The listing builds one solid part. Answer for the finished solid, in the listing's coordinates (mm). Face numbers are marked on the shaded views. Round coordinates to 2 decimals unless told otherwise and drop trailing zeros. Order: outer loops, then holes, each group sorted by start corner. A loop starts at its lowest first (then second) coordinate and runs counter-clockwise, first axis right, second up. Notation, with made-up numbers: (-39, 29.25) -> (-31, 29.25) arc R19 cw to (-31, 49.25) -> close; hole circle Ø11 at (36, -2). An arc over 180 degrees is marked (long way). Return JSON: item names as keys, results as strings. Group by question number.
(1) Each of these flat-tipped pins is pushed along its axis until it touches: pin 1 (2 mm diameter, centred on x = 0, y = 3, fed in from +Z); pin 2 (2.5 mm diameter, centred on x = -22.65, z = 16.46, fed in from -Y); pin 3 (5 mm diameter, centred on x = 19.02, z = 6.18, fed in from -Y); pin 4 (3 mm diameter, centred on x = -9, z = -26, fed in from -Y). Where does it stop, or does it pass through?
(2) The part is cut by section A-A (x = 0). Determine the outline of the cut face in (y, z), plus the area to 3 significant figures.
(3) Consider line 1 (Z direction, x = 0, y = 6.8); line 2 (Z direction, x = 23, y = 0.5); line 3 (X direction, y = 1, z = 25.5). Determine where each line is inside the solid, lowest interval first. Write a range as [from, to].
(4) The part is cut by section B-B (z = 0). Determine the outline of the cut face in (x, y), plus the area to 3 significant figures.
(5) Determine the mould class of the marked faces 1, 2 and 3 for opening direction X: +X half, -X half, draft (parallel to the pull), parting line (faces both ways), or undercut.
(6) The part is cut by section C-C (x = 28). Determine the outline of the cut face in (y, z), plus the area to 3 significant figures.
(7) The part is cut by section D-D (z = -8). Determine the outline of the cut face in (x, y).
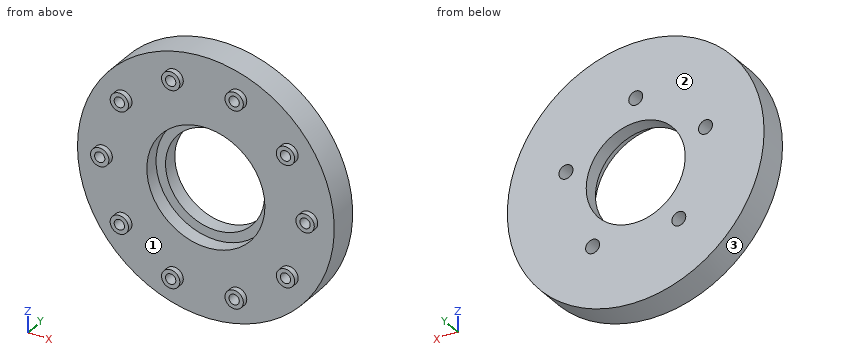
Autodesk Inventor part; units mm, degrees
ref_plane "YZ Plane" through (0, 0, 0) normal (1, 0, 0) x (0, 1, 0)
ref_plane "XZ Plane" through (0, 0, 0) normal (0, 1, 0) x (-1, 0, 0)
ref_plane "XY Plane" through (0, 0, 0) normal (0, 0, 1) x (1, 0, 0)
sketch "Szkic1" plane through (0, 0, 0) normal (0, 1, 0) x (-1, 0, 0)
  circle A0 centre (0, 0) radius 35
  dimension "d0" = 70
extrude "Wyciągnięcie proste1" add sketch "Szkic1" along normal blind 8
sketch "Szkic2" plane through (0, 0, 0) normal (0, -1, 0) x (1, 0, 0)
  circle A0 centre (0, 0) radius 28
  circle A1 centre (28, 0) radius 2.5
  dimension "d3" = 56
  dimension "d4" = 5
sketch "Szkic3" plane through (0, 0, 0) normal (0, -1, 0) x (1, 0, 0)
  circle A0 centre (0, 0) radius 16.1
  dimension "d9" = 32.2
extrude "Wyciągnięcie proste2" cut sketch "Szkic3" against normal blind 4
extrude "Wyciągnięcie proste3" add sketch "Szkic2" along normal blind 1.5 contours A0 A1 | A0 A1 picked at (27.2137, -0.5653) picked at (28.742, -0.6489)
pattern_circular "Szyk kołowy1" count 10 over 360 about axis through (0, 0, 0) along (0, 1, 0) of "Wyciągnięcie proste3"
sketch "Szkic4" plane through (0, 4, 0) normal (0, -1, 0) x (1, 0, 0)
  circle A0 centre (0, 0) radius 13.5
  dimension "d17" = 27
extrude "Wyciągnięcie proste4" cut sketch "Szkic4" against normal blind 4
sketch "Szkic5" plane through (28, -1.5, 0) normal (0, -1, 0) x (1, 0, 0)
  circle A0 centre (0, 0) radius 2.5
  circle A1 centre (0, 0) radius 1.4
  point P0 (-28, 0)
  dimension "d20" = 2.8
extrude "Wyciągnięcie proste5" cut sketch "Szkic5" against normal blind 6 contours A1
pattern_circular "Szyk kołowy2" count 10 over 360 about axis through (0, 0, 0) along (0, 1, 0) of "Wyciągnięcie proste5"
sketch "Szkic6" plane through (0, 8, 0) normal (0, 1, 0) x (1, 0, 0)
  circle A0 centre (0, 0) radius 20
  circle A1 centre (0, -20) radius 1.9
  dimension "d26" = 40
  dimension "d27" = 3.8
extrude "Wyciągnięcie proste6" cut sketch "Szkic6" against normal blind 6 contours A1 A0 | A0 A1 picked at (0.074, -19.3643) picked at (0.0625, -20.6235)
pattern_circular "Szyk kołowy3" count 5 over 360 about axis through (0, 4, 0) along (0, 1, 0) of "Wyciągnięcie proste6"
properties part number "_Drukowanie 3D"
Answer below:
{
 "1": {"pin 1": "stops at z = 35", "pin 2": "stops at y = 4.5", "pin 3": "stops at y = 0", "pin 4": "stops at y = -1.5"},
 "2": {"outline": "(0, -35) -> (8, -35) -> (8, -13.5) -> (4, -13.5) -> (4, -16.1) -> (0, -16.1) -> close; (0, 16.1) -> (4, 16.1) -> (4, 13.5) -> (8, 13.5) -> (8, 18.1) -> (2, 18.1) -> (2, 21.9) -> (8, 21.9) -> (8, 35) -> (0, 35) -> close", "area": "300 mm²"},
 "3": {"line 1": "z = [-35, -13.5], [13.5, 18.1], [21.9, 35]", "line 2": "z = [-26.38, -17.81], [-15.1, 15.1], [17.81, 26.38]", "line 3": "x = [-23.97, -9.48], [-7.83, 7.83], [9.48, 23.97]"},
 "4": {"outline": "(-35, 0) -> (-30.5, 0) -> (-30.5, -1.5) -> (-29.4, -1.5) -> (-29.4, 4.5) -> (-26.6, 4.5) -> (-26.6, -1.5) -> (-25.5, -1.5) -> (-25.5, 0) -> (-16.1, 0) -> (-16.1, 4) -> (-13.5, 4) -> (-13.5, 8) -> (-35, 8) -> close; (13.5, 4) -> (16.1, 4) -> (16.1, 0) -> (25.5, 0) -> (25.5, -1.5) -> (26.6, -1.5) -> (26.6, 4.5) -> (29.4, 4.5) -> (29.4, -1.5) -> (30.5, -1.5) -> (30.5, 0) -> (35, 0) -> (35, 8) -> (13.5, 8) -> close", "area": "305 mm²"},
 "5": {"face 1": "undercut", "face 2": "draft", "face 3": "parting line"},
 "6": {"outline": "(-1.5, -2.5) -> (0, -2.5) -> (0, -21) -> (8, -21) -> (8, 21) -> (0, 21) -> (0, 2.5) -> (-1.5, 2.5) -> (-1.5, 1.4) -> (4.5, 1.4) -> (4.5, -1.4) -> (-1.5, -1.4) -> close", "area": "327 mm²"},
 "7": {"outline": "(-34.07, 0) -> (-13.97, 0) -> (-13.97, 4) -> (-10.87, 4) -> (-10.87, 8) -> (-34.07, 8) -> close; (10.87, 4) -> (13.97, 4) -> (13.97, 0) -> (34.07, 0) -> (34.07, 8) -> (10.87, 8) -> close"}
}
